Check sheet for the modelled part. Datum: model origin and axes. Units: mm. Round coordinates to 2 decimals unless told otherwise and drop trailing zeros. Write each loop counter-clockwise with the first axis right and the second up, starting at its lowest first coordinate (ties: lowest second). Pieces come first, ordered by that corner, then holes. Notation, with made-up numbers: (67, -26) -> (123, -26) arc R25 cw to (123, -13) -> close; hole circle Ø3 at (27, -37.75). An arc over 180 degrees is marked (long way). One line per item, written item: value.
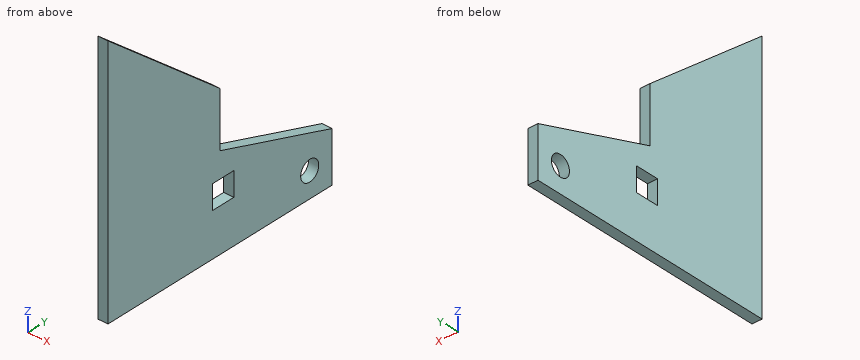
from build123d import *

# Parameters (mm, degrees)
SKETCH1_R           = 6.05
SKETCH1_W           = 14.2
SKETCH1_H           = 14.2
BOSS_EXTRUDE1_DEPTH = 6


with BuildPart() as part:
    # Sketch1 → Boss-Extrude1 (new body)
    with BuildSketch(Plane(origin=(0, 0, 0), x_dir=(0, 0, -1), z_dir=(1, 0, 0))):
        Polygon((-150, 0), (-88, 75), (-55, 75), (-30, 150), (0, 150), (0, 0), align=None)
        with Locations((-15, 135)):
            Circle(SKETCH1_R, mode=Mode.SUBTRACT)
        with Locations((-32.9, 77.1)):
            Rectangle(SKETCH1_W, SKETCH1_H, mode=Mode.SUBTRACT)
    extrude(amount=BOSS_EXTRUDE1_DEPTH)


solid = part.part
Item 1: Sectioned sample at B-B (y = 135). Enter the section's corners in (x, z), then the cut area to 3 significant figures.
Result set:
outline: (0, 0) -> (6, 0) -> (6, 8.95) -> (0, 8.95) -> close; (0, 21.05) -> (6, 21.05) -> (6, 35) -> (0, 35) -> close
area: 137 mm^2
Item 2: Sectioned sample at A-A (z = 15). Enter the section's corners in (x, y), then the cut area to 3 significant figures.
Result set:
outline: (0, 0) -> (6, 0) -> (6, 128.95) -> (0, 128.95) -> close; (0, 141.05) -> (6, 141.05) -> (6, 150) -> (0, 150) -> close
area: 827 mm^2
Item 3: Depth check by flat-ended pin: pin 1 (8 mm diameter, centred on y = 56.5, z = 42.5, fed in from -X); pin 2 (1.8 mm diameter, centred on x = 3, z = 76, fed in from +Y); pin 3 (2 mm diameter, centred on x = 4, z = 109.5, fed in from +Y); pin 4 (1.5 mm diameter, centred on x = 5, z = 94, fed in from +Y). Enter the tip coordinate at first touch or a pass-through.
Result set:
pin 1: x = 0
pin 2: y = 75
pin 3: y = 50.2
pin 4: y = 68.65
Item 4: Material ranges on line 1 along Y through (x, z) = (2.3, 15); line 2 along Z through (x, y) = (0.9, 83); line 3 along Y through (x, z) = (2.7, 68.5), recorded low to high.
Result set:
line 1: 0 to 128.95, 141.05 to 150
line 2: 0 to 25.8, 40 to 52.33
line 3: 0 to 75
Item 5: Sectioned sample at D-D (z = 119). Enter the section's corners in (x, y), then the cut area to 3 significant figures.
Result set:
outline: (0, 0) -> (6, 0) -> (6, 37.5) -> (0, 37.5) -> close
area: 225 mm^2
Item 6: Sectioned sample at C-C (x = 2.3). Enter the section's corners in (y, z), then the cut area to 3 significant figures.
Result set:
outline: (0, 0) -> (150, 0) -> (150, 30) -> (75, 55) -> (75, 88) -> (0, 150) -> close; hole (70, 25.8) -> (84.2, 25.8) -> (84.2, 40) -> (70, 40) -> close; hole circle Ø12.1 at (135, 15)
area: 11,800 mm^2
